```python
from build123d import *

# Parameters (mm, degrees)
SKETCH_1_R          = 6.5
SKETCH_1_R_2        = 1.5
EXTRUDE_1_DEPTH     = 3
SKETCH_2_W          = 40
SKETCH_2_H          = 3
EXTRUDE_2_DEPTH     = 44
FILLET_4_R          = 3
SKETCH_3_R          = 2
CUT_EXTRUDE_1_DEPTH = 77.974021592
FILLET_5_R          = 3
FILLET_6_R          = 3


with BuildPart() as part:
    # Эскиз1 → Бобышка-Вытянуть1 (new body)
    with BuildSketch(Plane.XY):
        with BuildLine():
            Line((0, 0), (40, 0))
            Line((40, 0), (40, 26))
            ThreePointArc((40, 26), (20, 46), (0, 26))
            Line((0, 26), (0, 0))
        make_face()
        with Locations((20, 26)):
            Circle(SKETCH_1_R, mode=Mode.SUBTRACT)
        with Locations((32.5, 26)):
            Circle(SKETCH_1_R_2, mode=Mode.SUBTRACT)
        with Locations((7.5, 26)):
            Circle(SKETCH_1_R_2, mode=Mode.SUBTRACT)
    extrude(amount=EXTRUDE_1_DEPTH)

    # Эскиз2 → Бобышка-Вытянуть2 (add)
    with BuildSketch(Plane.XY.offset(3)):
        with Locations((20, 1.5)):
            Rectangle(SKETCH_2_W, SKETCH_2_H)
    extrude(amount=EXTRUDE_2_DEPTH)

    # Скругление4
    fillet_4_edges = [part.edges().sort_by_distance(p)[0] for p in [
        (20, 0, 0),
    ]]
    fillet(fillet_4_edges, radius=FILLET_4_R)

    # Эскиз3 → Вырез-Вытянуть1 (cut, through all)
    with BuildSketch(Plane.XZ):
        with Locations(Location((5, 37, 0), (0, 0, 270))):
            Circle(SKETCH_3_R)
        with Locations(Location((35, 37, 0), (0, 0, 270))):
            Circle(SKETCH_3_R)
        with Locations(Location((5, 13, 0), (0, 0, 270))):
            Circle(SKETCH_3_R)
        with Locations(Location((35, 13, 0), (0, 0, 270))):
            Circle(SKETCH_3_R)
    extrude(amount=-CUT_EXTRUDE_1_DEPTH, mode=Mode.SUBTRACT)

    # Скругление5
    fillet_5_edges = [part.edges().sort_by_distance(p)[0] for p in [
        (20, 3, 3),
    ]]
    fillet(fillet_5_edges, radius=FILLET_5_R)

    # Скругление6
    fillet_6_edges = [part.edges().sort_by_distance(p)[0] for p in [
        (40, 1.5, 47),
        (0, 1.5, 47),
    ]]
    fillet(fillet_6_edges, radius=FILLET_6_R)


solid = part.part
```
Could you check a few things on this model? Use its own coordinates, in mm. A direction names the side the tool comes from. Coordinates: 2 decimals unless noted, no trailing zeros. Write each loop counter-clockwise with the first axis right and the second up, starting at its lowest first coordinate (ties: lowest second). Pieces come first, ordered by that corner, then holes. Notation, with made-up numbers: (-28, -12.5) -> (-3, -12.5) arc R21 ccw to (-3, 15.5) -> close; hole circle Ø11 at (-24, -17.75). An arc over 180 degrees is marked (long way). Write item = value, one per line. Start each with the question number.
(1) I want a section at D-D (y = 21). Please give me the cut outline in (x, z), plus the area to 3 significant figures.
(2) We'd pull the mould along Z, two halves only. Please class faces 1 (the face through (20.28, 3.9, 3.86)), 2 (the face through (20, 3, 26)), 3 (the face through (5, 1, 39)), 4 (the face through (15, 20, 0)): released by +Z, released by -Z, zero draft, split by the parting line, or undercut.
(3) I need wall thicknesses on line 1 (X direction, y = 2, z = 37); line 2 (Y direction, x = 19.5, z = 27.5). Which ranges of each line are inside material? Lowest first, please. Write a range as [from, to].
(4) I want a section at C-C (y = 29). Please give me the cut outline in (x, z).
(5) I want a section at B-B (x = 20). Please give me the cut outline in (y, z), plus the area to 3 significant figures.
(6) Will these pins go through, and if not, where does the flat tip stop? pin 1 (10 mm diameter, centred on y = 29, z = 9.5, fed in from -X); pin 2 (5 mm diameter, centred on x = 5, z = 37, fed in from +Y); pin 3 (3.5 mm diameter, centred on x = 32.5, y = 26, fed in from +Z).
(7) I want a section at A-A (z = 13). Please give me the cut outline in (x, y).
(8) Which directions (+Z, -Z, +X, -X, +Y, -Y) give clear straight access to the entire face, cutting with the end or side of a thin tool? Please do faces 5 (the face through (39.1, 1.52, 46.14)), 6 (the face through (20, 17, 3)).
Result set:
q1.outline = (0, 0) -> (15.85, 0) -> (15.85, 3) -> (0, 3) -> close; (24.15, 0) -> (40, 0) -> (40, 3) -> (24.15, 3) -> close
q1.area = 95.1 mm2
q2.face_1 = released by +Z
q2.face_2 = zero draft
q2.face_3 = undercut
q2.face_4 = released by -Z
q3.line_1 = [0, 3], [7, 33], [37, 40]
q3.line_2 = [0, 3]
q4.outline = (0.23, 0) -> (14.23, 0) -> (14.23, 3) -> (0.23, 3) -> close; (25.77, 0) -> (39.77, 0) -> (39.77, 3) -> (25.77, 3) -> close
q5.outline = (0, 3) arc R3 ccw to (3, 0) -> (19.5, 0) -> (19.5, 3) -> (6, 3) arc R3 cw to (3, 6) -> (3, 47) -> (0, 47) -> close; (32.5, 0) -> (46, 0) -> (46, 3) -> (32.5, 3) -> close
q5.area = 231 mm2
q6.pin_1 = through
q6.pin_2 = 3
q6.pin_3 = 3
q7.outline = (0, 0) -> (3, 0) -> (3, 3) -> (0, 3) -> close; (7, 0) -> (33, 0) -> (33, 3) -> (7, 3) -> close; (37, 0) -> (40, 0) -> (40, 3) -> (37, 3) -> close
q8.face_5 = +Z, +X, +Y, -Y
q8.face_6 = +Z, +X, -X, +Y
